Source: CAD feature listing. Evaluate the final solid. Frame: model axes, mm. Face numbers are marked on the shaded views. Coordinates: 2 decimals unless noted, no trailing zeros. Order: outer loops, then holes, each group sorted by start corner. A loop starts at its lowest first (then second) coordinate and runs counter-clockwise, first axis right, second up.
Autodesk Inventor part; units mm, degrees
ref_plane "YZ Plane" through (0, 0, 0) normal (1, 0, 0) x (0, 1, 0)
ref_plane "XZ Plane" through (0, 0, 0) normal (0, 1, 0) x (-1, 0, 0)
ref_plane "XY Plane" through (0, 0, 0) normal (0, 0, 1) x (1, 0, 0)
sketch "草圖1" plane through (0, 0, 0) normal (0, 0, 1) x (1, 0, 0)
  line L0 (-1, 2.5) -> (1, 2.5)
  line L1 (1, 2.5) -> (1, -2.5)
  line L2 (1, -2.5) -> (-1, -2.5)
  line L3 (-1, -2.5) -> (-1, 2.5)
  line L4 (-1, 2.5) -> (1, -2.5) construction
  line L5 (1, 2.5) -> (-1, -2.5) construction
  line L6 (-0.8, -0.1) -> (0.8, -0.1)
  line L7 (1, -0.1) -> (1, 0.1)
  line L8 (0.8, 0.1) -> (-0.8, 0.1)
  line L9 (-1, 0.1) -> (-1, -0.1)
  line L10 (-1, -0.1) -> (1, 0.1) construction
  line L11 (1, -0.1) -> (-1, 0.1) construction
  line L12 (-0.8, -2.3) -> (0.8, -2.3)
  line L13 (0.8, 2.3) -> (-0.8, 2.3)
  line L14 (-0.8, 2.3) -> (0.8, -2.3) construction
  line L15 (-0.8, -2.3) -> (0.8, 2.3) construction
  line L16 (0.8, -2.3) -> (0.8, -0.08)
  line L17 (0.8, 0.08) -> (0.8, 2.3)
  line L18 (-0.8, 2.3) -> (-0.8, 0.08)
  line L19 (-0.8, -0.08) -> (-0.8, -2.3)
  line L20 (-1, -2.5) -> (1, -2.5)
  line L21 (1, -2.5) -> (1, -5.5)
  line L22 (1, -5.5) -> (-1, -5.5)
  line L23 (-1, -5.5) -> (-1, -2.5)
  line L24 (-0.9, -2.4) -> (0.9, -2.4)
  line L25 (0.9, -2.4) -> (0.9, 2.4)
  line L26 (0.9, 2.4) -> (-0.9, 2.4)
  line L27 (-0.9, 2.4) -> (-0.9, -2.4)
  line L28 (-0.9, -2.4) -> (0.9, 2.4) construction
  line L29 (0.9, -2.4) -> (-0.9, 2.4) construction
  point P0 (0, 0)
  dimension "d0" = 2
  dimension "d1" = 5
  dimension "d4" = 0.2
  dimension "d5" = 4.6
  dimension "d6" = 1.6
  dimension "d7" = 3
  dimension "d12" = 1.8
  dimension "d13" = 4.8
extrude "擠出4" add sketch "草圖1" along normal blind 0.6 contours L0 L1 L2 L3
extrude "擠出5" add sketch "草圖1" along normal blind 0.55 contours L27 L26 L25 L24
extrude "擠出6" add sketch "草圖1" along normal blind 0.5 contours L2 L21 L22 L23 | L6 L16 L12 L19 | L8 L18 L13 L17
properties part number "窗" material "木材 (胡桃木)"
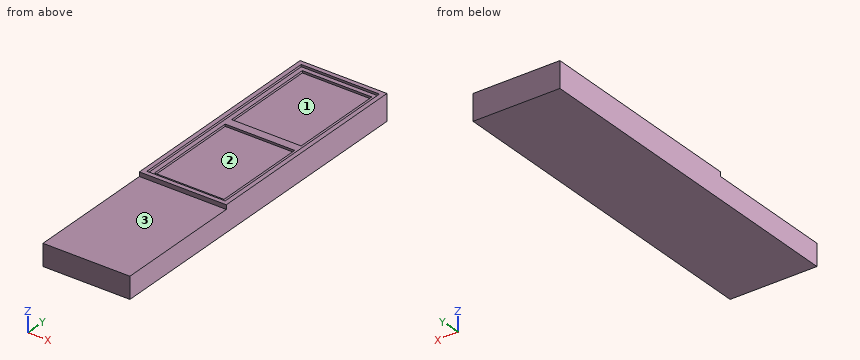
Q1. Pull-direction query (X, two-part tool) for the marked faces 1, 2 and 3; classes: pulls with the +X half, pulls with the -X half, needs draft (parallel to the pull), parting line crosses it, or undercut.
Solutions:
face 1: undercut
face 2: undercut
face 3: needs draft
Q2. Section query C-C on y = -3.25. Output: boundary loops of the cut face in (x, z).
Solutions:
outline: (-1, 0) - (1, 0) - (1, 0.5) - (-1, 0.5) - close
Q3. Section query A-A on y = -1.25. Output: boundary loops of the cut face in (x, z).
Solutions:
outline: (-1, 0) - (1, 0) - (1, 0.6) - (0.9, 0.6) - (0.9, 0.55) - (0.8, 0.55) - (0.8, 0.5) - (-0.8, 0.5) - (-0.8, 0.55) - (-0.9, 0.55) - (-0.9, 0.6) - (-1, 0.6) - close
Q4. Material intervals for line 1 along Z through (x, y) = (-0.75, -3.5); line 2 along Z through (x, y) = (-0.85, -1.75), sorted ascending.
Solutions:
line 1: z = 0 to 0.5
line 2: z = 0 to 0.55
Q5. Pin query (flat end, axial travel): P1, Ø0.5, axis at x = 0, y = 0.5, coming from the +Z side. Return the tip coordinate at first contact, or that it passes through.
Solutions:
P1: stops at z = 0.5
Q6. Section query B-B on x = 0.4. Output: boundary loops of the cut face in (y, z).
Solutions:
outline: (-5.5, 0) - (2.5, 0) - (2.5, 0.6) - (2.4, 0.6) - (2.4, 0.55) - (2.3, 0.55) - (2.3, 0.5) - (0.1, 0.5) - (0.1, 0.55) - (-0.1, 0.55) - (-0.1, 0.5) - (-2.3, 0.5) - (-2.3, 0.55) - (-2.4, 0.55) - (-2.4, 0.6) - (-2.5, 0.6) - (-2.5, 0.5) - (-5.5, 0.5) - close
